from build123d import *

# Parameters (mm, degrees)
F0_W     = 378.75718
F0_H     = 914.4
F1_DEPTH = 12.7
F3_DEPTH = 12.701
F4_W     = 203.2
F4_H     = 25.4
F5_DEPTH = 25.4


with BuildPart() as f1:
    # F0 (on Top) → F1 (new body)
    with BuildSketch(Plane.XY):
        with Locations((-4.136321, 70.025934)):
            Rectangle(F0_W, F0_H)
    extrude(amount=F1_DEPTH)

    # F2 (on face) → F3 (cut, through all)
    with BuildSketch(Plane.XY.offset(12.7)):
        with BuildLine():
            Line((-142.714911, 514.525934), (-142.714911, 511.350934))
            ThreePointArc((-142.714911, 511.350934), (-140.469847, 512.28087), (-139.539911, 514.525934))
            ThreePointArc((-139.539911, 514.525934), (-140.469847, 516.770998), (-142.714911, 517.700934))
            Line((-142.714911, 517.700934), (-142.714911, 514.525934))
        make_face()
        with BuildLine():
            ThreePointArc((-142.714911, 517.700934), (-145.889911, 514.525934), (-142.714911, 511.350934))
            Line((-142.714911, 511.350934), (-142.714911, 514.525934))
            Line((-142.714911, 514.525934), (-142.714911, 517.700934))
        make_face()
        with BuildLine():
            Line((134.442269, 514.525934), (134.442269, 511.350934))
            ThreePointArc((134.442269, 511.350934), (136.687333, 512.28087), (137.617269, 514.525934))
            ThreePointArc((137.617269, 514.525934), (136.687333, 516.770998), (134.442269, 517.700934))
            Line((134.442269, 517.700934), (134.442269, 514.525934))
        make_face()
        with BuildLine():
            ThreePointArc((134.442269, 517.700934), (131.267269, 514.525934), (134.442269, 511.350934))
            Line((134.442269, 511.350934), (134.442269, 514.525934))
            Line((134.442269, 514.525934), (134.442269, 517.700934))
        make_face()
        with BuildLine():
            ThreePointArc((-142.714911, -377.649066), (-140.469847, -376.71913), (-139.539911, -374.474066))
            ThreePointArc((-139.539911, -374.474066), (-144.959975, -372.229002), (-142.714911, -377.649066))
        make_face()
        with BuildLine():
            ThreePointArc((134.442269, -377.649066), (136.687333, -376.71913), (137.617269, -374.474066))
            ThreePointArc((137.617269, -374.474066), (136.687333, -372.229002), (134.442269, -371.299066))
            Line((134.442269, -371.299066), (134.442269, -374.474066))
            Line((134.442269, -374.474066), (134.442269, -377.649066))
        make_face()
        with BuildLine():
            Line((134.442269, -374.474066), (134.442269, -371.299066))
            ThreePointArc((134.442269, -371.299066), (131.267269, -374.474066), (134.442269, -377.649066))
            Line((134.442269, -377.649066), (134.442269, -374.474066))
        make_face()
    extrude(amount=-F3_DEPTH, mode=Mode.SUBTRACT)

    # F4 (on face) → F5 (cut)
    with BuildSketch(Plane.XY.offset(12.7)):
        with Locations((-9.051421, 376.754831)):
            Rectangle(F4_W, F4_H)
        with Locations((-9.051421, -268.405143)):
            Rectangle(F4_W, F4_H)
    extrude(amount=-F5_DEPTH, mode=Mode.SUBTRACT)


solid = f1.part
Work out the finished part from the listing and answer in its coordinate system (mm). Give positions to 0.01 mm unless a question says otherwise; leave off trailing zeros. Order: outer loops, then holes, each group sorted by start corner. A loop starts at its lowest first (then second) coordinate and runs counter-clockwise, first axis right, second up. Notation, with made-up numbers: (-38, -13) - (12, -13) arc R27 ccw to (12, 4) - close; hole circle Ø2 at (61, 55.25). An arc over 180 degrees is marked (long way). Answer as CSV lines item,"result". Start each with the question number.
Q1. The part is cut by section A-A (x = 4). Write down the section's boundary in (y, z).
Q2. Given pin 1 Ø12 at (x, y) = (59.5, 64.5) entering from -Z, flat-ended and moving along its own axis, determine where the tip first touches the part or whether it passes through.
Q3. The part is cut by section B-B (z = 10.75). Write down the section's boundary in (x, y) (3 decimals), then the cut area to 3 significant figures.
Q4. Find the intervals of material crossed by L1, parallel to Y at x = 80, z = 3.5; L2, parallel to X at y = -272, z = 12, in increasing order. Write a range as [from, to].
Check result:
1,outline,"(-387.17, 0) - (-281.11, 0) - (-281.11, 12.7) - (-387.17, 12.7) - close; (-255.71, 0) - (364.05, 0) - (364.05, 12.7) - (-255.71, 12.7) - close; (389.45, 0) - (527.23, 0) - (527.23, 12.7) - (389.45, 12.7) - close"
2,pin 1,"stops at z = 0"
3,outline,"(-193.515, -387.174) - (185.242, -387.174) - (185.242, 527.226) - (-193.515, 527.226) - close; hole circle Ø6.35 at (-142.715, -374.474); hole circle Ø6.35 at (-142.715, 514.526); hole (-110.651, -281.105) - (92.549, -281.105) - (92.549, -255.705) - (-110.651, -255.705) - close; hole (-110.651, 364.055) - (92.549, 364.055) - (92.549, 389.455) - (-110.651, 389.455) - close; hole circle Ø6.35 at (134.442, -374.474); hole circle Ø6.35 at (134.442, 514.526)"
3,area,"336,000 mm²"
4,L1,"y = [-387.17, -281.11], [-255.71, 364.05], [389.45, 527.23]"
4,L2,"x = [-193.51, -110.65], [92.55, 185.24]"
